Could you check a few things on this drawing? It's one solid part, dimensions in mm from its lowest x, y, z. A direction names the side the tool comes from. Coordinates: 2 decimals unless noted, no trailing zeros. Write each loop counter-clockwise with the first axis right and the second up, starting at its lowest first coordinate (ties: lowest second). Pieces come first, ordered by that corner, then holes.
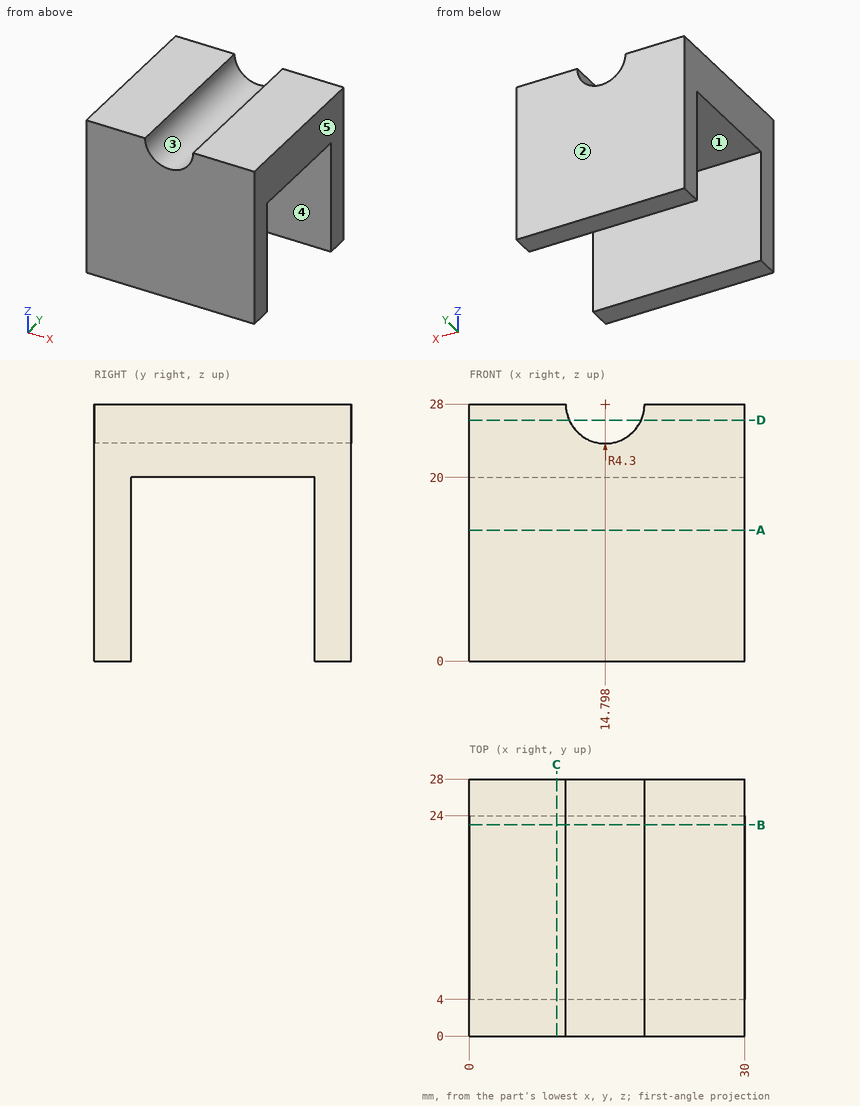
1) Imagine slicing it at D-D on z = 26.25. Please give me the cut outline in (x, y) (1 decimal), then the cut area to 3 significant figures.
Values follow:
outline: (0, 0) - (10.9, 0) - (10.9, 28) - (0, 28) - close; (18.7, 0) - (30, 0) - (30, 28) - (18.7, 28) - close
area: 620 mm2
2) Imagine slicing it at C-C on x = 9.5. Please give me the cut outline in (y, z).
Values follow:
outline: (0, 0) - (4, 0) - (4, 20) - (24, 20) - (24, 0) - (28, 0) - (28, 28) - (0, 28) - close
3) On a 3-axis mill with a long thin cutter (end or side, diameter ignored), from which of +Z, -Z, +X, -X, +Y, -Y can I reach the whole of each face in a straight line? I mean the marked faces 4 and 5. Say none if no direction works.
Values follow:
face 4: -Z, +X, -X
face 5: +Z, -Z, +X, +Y, -Y
4) Will this pin go through, and if not, where does the flat tip stop? pin 1 (1 mm diameter, centred on x = 13, y = 16.5, fed in from -Z).
Values follow:
pin 1: stops at z = 20
5) Imagine slicing it at A-A on z = 14.25. Please give me the cut outline in (x, y).
Values follow:
outline: (0, 0) - (30, 0) - (30, 4) - (0, 4) - close; (0, 24) - (30, 24) - (30, 28) - (0, 28) - close
6) We'd pull the mould along Y, two halves only. Please class the marked faces 1, 2 and 3: pulls with the +Y half, pulls with the -Y half, needs draft (parallel to the pull), parting line crosses it, or undercut.
Values follow:
face 1: undercut
face 2: pulls with the +Y half
face 3: needs draft
7) I need wall thicknesses on probe 1 along Y at (x, z) = (14, 5.25); probe 2 along Z at (x, y) = (26.25, 11); probe 3 along X at (y, z) = (16.75, 25.25) (1 decimal). Which ranges of each line are inside material? Lowest first, please.
Values follow:
probe 1: y = 0 to 4, 24 to 28
probe 2: z = 20 to 28
probe 3: x = 0 to 11.5, 18.1 to 30
8) Imagine slicing it at B-B on y = 23. Please give me the cut outline in (x, z).
Values follow:
outline: (0, 20) - (30, 20) - (30, 28) - (19.1, 28) arc R4.3 cw to (10.5, 28) - (0, 28) - close
